Geometry: see drawing. Coordinates: mm, zero at the bounding-box minimum. A direction names the side the tool comes from. Give positions to 0.01 mm unless a question says otherwise; leave off trailing zeros. Loops run counter-clockwise (first coordinate to the right, second up) from the corner with the lowest first, then second, coordinate; pieces in that order, holes last. Notation, with made-up numbers: (66.5, 29) -> (111.5, 29) arc R6 ccw to (111.5, 40) -> close; hole circle Ø3 at (15.25, 51). An arc over 180 degrees is marked (long way). Use CSV: the item, a comma, the result in double quotes.
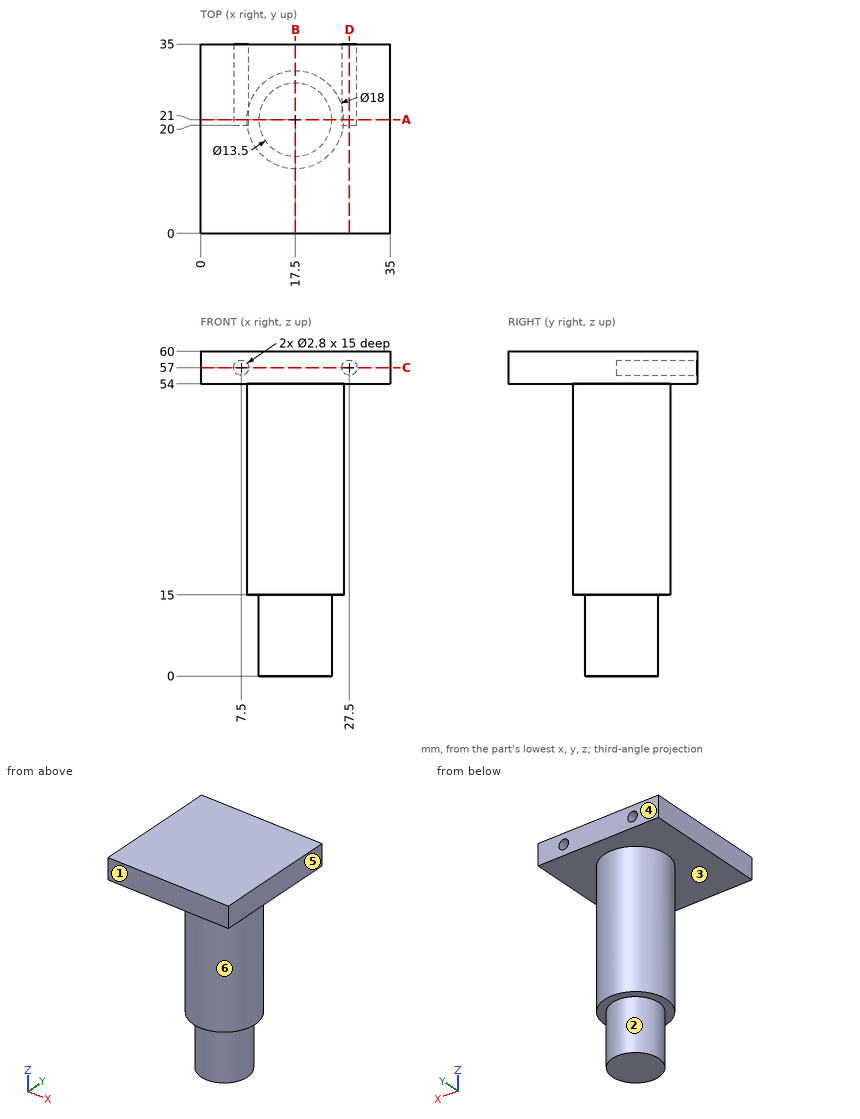
1) Mould query, pull axis Y, two halves, no side actions, for the marked faces 1, 2, 3 and 4. Classes: pulls with the +Y half, pulls with the -Y half, needs draft (parallel to the pull), parting line crosses it, or undercut.
From the geometry:
face 1,"pulls with the -Y half"
face 2,"parting line crosses it"
face 3,"needs draft"
face 4,"pulls with the +Y half"
2) Contact query for flat-ended pins moving along their axis: pin 1 (1.7 mm diameter, centred on x = 7.5, z = 57, fed in from +Y); pin 2 (2 mm diameter, centred on y = 27, z = 44.5, fed in from -X); pin 3 (10 mm diameter, centred on x = 30.5, y = 7, fed in from -Z). Output: stop coordinate, or through.
From the geometry:
pin 1,"stops at y = 20"
pin 2,"stops at x = 10.02"
pin 3,"stops at z = 54"
3) Ray query, line 1 (X direction, y = 27, z = 57); line 2 (Z direction, x = 7.5, y = 28); line 3 (Z direction, x = 5, y = 4). Return the intervals inside material, ascending.
From the geometry:
line 1,"x = 0 to 6.1, 8.9 to 26.1, 28.9 to 35"
line 2,"z = 54 to 55.6, 58.4 to 60"
line 3,"z = 54 to 60"
4) Section query D-D (x = 27.5). Return loops of the section in (y, z), then the cut area to 3 significant figures.
From the geometry:
outline,"(0, 54) -> (35, 54) -> (35, 55.6) -> (20, 55.6) -> (20, 58.4) -> (35, 58.4) -> (35, 60) -> (0, 60) -> close"
area,"168 mm^2"
5) Reachability of the marked faces 5 and 6 from +Z, -Z, +X, -X, +Y, -Y: full face, straight path, thin tool, end or side. Return the list, or none.
From the geometry:
face 5,"+Z, -Z, +X, +Y, -Y"
face 6,"-Z"
6) Section query B-B (x = 17.5). Return loops of the section in (y, z), then the cut area to 3 significant figures.
From the geometry:
outline,"(0, 54) -> (12, 54) -> (12, 15) -> (14.25, 15) -> (14.25, 0) -> (27.75, 0) -> (27.75, 15) -> (30, 15) -> (30, 54) -> (35, 54) -> (35, 60) -> (0, 60) -> close"
area,"1,110 mm^2"
7) Section query C-C (z = 57). Return loops of the section in (x, y), then the cut area to 3 significant figures.
From the geometry:
outline,"(0, 0) -> (35, 0) -> (35, 35) -> (28.9, 35) -> (28.9, 20) -> (26.1, 20) -> (26.1, 35) -> (8.9, 35) -> (8.9, 20) -> (6.1, 20) -> (6.1, 35) -> (0, 35) -> close"
area,"1,140 mm^2"
8) Section query A-A (y = 21). Return loops of the section in (x, z).
From the geometry:
outline,"(0, 54) -> (8.5, 54) -> (8.5, 15) -> (10.75, 15) -> (10.75, 0) -> (24.25, 0) -> (24.25, 15) -> (26.5, 15) -> (26.5, 54) -> (35, 54) -> (35, 60) -> (0, 60) -> close; hole circle Ø2.8 at (7.5, 57); hole circle Ø2.8 at (27.5, 57)"
